The listing builds one solid part. Answer for the finished solid, in the listing's coordinates (mm). Coordinates: 2 decimals unless noted, no trailing zeros. Order: outer loops, then holes, each group sorted by start corner. A loop starts at its lowest first (then second) coordinate and runs counter-clockwise, first axis right, second up.
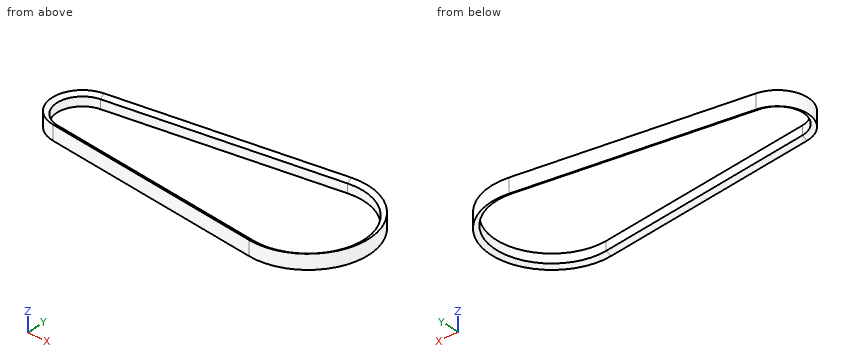
Autodesk Inventor part; units mm, degrees
ref_plane "Work Plane1" through (-3.0593, 22.7956, 0) normal (-0.9911143, -0.1330127, 0) x (0.1330127, -0.9911143, 0)
ref_plane "YZ Plane" through (0, 0, 0) normal (1, 0, 0) x (0, 1, 0)
ref_plane "XZ Plane" through (0, 0, 0) normal (0, 1, 0) x (-1, 0, 0)
sketch "Sketch1" plane through (0, 0, 0) normal (0, 0, 1) x (1, 0, 0)
  arc A0 (-3.0584, -22.7957) -> (-3.0593, 22.7956) centre (0, 0) ccw
  arc A1 (-95.3861, 10.4049) -> (-95.3857, -10.4086) centre (-93.9895, -0.0018) ccw
  line L0 (-95.3861, 10.4049) -> (-3.0593, 22.7956)
  line L1 (-95.3857, -10.4086) -> (-3.0584, -22.7957)
  dimension "d0" = 46
  dimension "d1" = 21
ref_plane "Work Plane1" through (-3.0593, 22.7956, 0) normal (-0.9911143, -0.1330127, 0) x (0.1330127, -0.9911143, 0)
sketch "Sketch2" plane through (-3.0593, 22.7956, 0) normal (-0.9911143, -0.1330127, 0) x (0.1330127, -0.9911143, 0)
  line L0 (-2, 0) -> (-2, 3)
  line L1 (-2, 0) -> (-2, -3)
  line L2 (-2, -3) -> (0, -1.8453)
  line L3 (0, -1.8453) -> (0, 1.8453)
  line L4 (0, 1.8453) -> (-2, 3)
  point P0 (23, 0)
  dimension "d4" = 3
  dimension "d5" = 3
  dimension "d6" = 60
  dimension "d7" = 60
  dimension "d8" = 2
sweep "Sweep1" add profiles "Sketch2" path "Sketch1"
properties part number "Dây đai"
(1) Given pin 1 Ø2 at (y, z) = (10, -1.5) entering from -X; pin 2 Ø2 at (x, y) = (-27.5, 19) entering from +Z, each flat-ended and moving along its own axis, determine where each tip first touches the part or whether it passes through.
(2) Find section B-B on x = -75. Determine the outline of the cut face in (y, z), then the cut area to 3 significant figures.
(3) Find the intervals of material crossed by probe 1 along Y at (x, z) = (-70.5, -2.5); probe 2 along Y at (x, z) = (-37.5, 0); probe 3 along X at (y, z) = (-8.5, 1.5), in increasing order.
(4) Find section A-A on z = -0.75. Determine the outline of the cut face in (x, y).
Resolved:
1. pin 1: stops at x = -102.66
1. pin 2: stops at z = 2.13
2. outline: (-15.16, -3) - (-13.14, -1.85) - (-13.14, 1.85) - (-15.16, 3) - close; (13.14, -1.85) - (15.16, -3) - (15.16, 3) - (13.14, 1.85) - close
2. area: 19.6 mm2
3. probe 1: y = -15.77 to -14.89, 14.89 to 15.76
3. probe 2: y = -20.19 to -18.17, 18.17 to 20.19
3. probe 3: x = -103.16 to -100.16, 21.37 to 23.51
4. outline: (-95.65, -12.39) - (-3.32, -24.78) arc R25 ccw (long way) to (-3.33, 24.78) - (-95.65, 12.39) arc R12.5 ccw to start; hole (-95.39, -10.41) - (-3.06, -22.8) arc R23 ccw (long way) to (-3.06, 22.8) - (-95.39, 10.4) arc R10.5 ccw to start
